Solid Edge part; units mm, degrees
sketch "Sketch1" plane through (0, 0, 0) normal (0, -1, 0) x (1, 0, 0)
  line L0 (0, 0) -> (-45, 0)
  line L1 (-45, 0) -> (-45, -4)
  line L2 (0, -4) -> (-45, -4)
  line L3 (28.2843, -32.2843) -> (0, -4)
  line L4 (30.2843, -30.2843) -> (28.2843, -32.2843)
  line L5 (0, 0) -> (30.2843, -30.2843)
  dimension "D1" = 45
  dimension "D2" = 28.2843
extrude "Protrusion1" add sketch "Sketch1" along normal mid plane 30
sketch "Sketch2" plane through (-15, 0, 0) normal (0, 0, 1) x (1, 0, 0)
  circle A0 centre (-8, 0) radius 7.5
  dimension "D1" = 8
extrude "Cutout1" cut sketch "Sketch2" against normal up to surface (4 mm away)
sketch "Sketch3" plane through (10.6066, 0, -10.6066) normal (0.7071068, 0, 0.7071068) x (0.7071068, 0, -0.7071068)
  circle A0 centre (10.8284, 0) radius 7.5
extrude "Cutout2" cut sketch "Sketch3" against normal up to surface (2.8284 mm away)
properties material "Stainless steel"
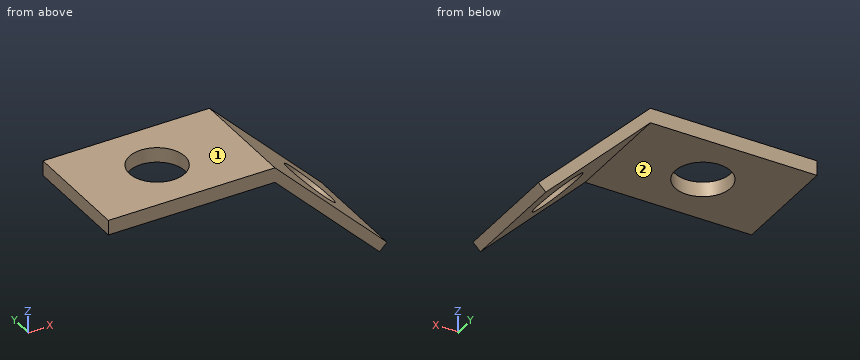
Can you work these out from the model? Positions are in its coordinate system, mm. Face numbers are marked on the shaded views. A direction names the side the tool comes from. Give positions to 0.01 mm unless a question says otherwise; leave off trailing zeros. Order: outer loops, then holes, each group sorted by start corner. A loop starts at its lowest first (then second) coordinate and runs counter-clockwise, first axis right, second up. Notation, with made-up numbers: (89, 55) - (93, 55) arc R32 cw to (93, 92) - close; hole circle Ø4 at (88.25, 38.5). An arc over 180 degrees is marked (long way). Use a Markdown table: item, result. Add a question column.
Q1. On a 3-axis mill with a long thin cutter (end or side, diameter ignored), from which of +Z, -Z, +X, -X, +Y, -Y can I reach the whole of each face in a straight line? I mean the marked faces 1 and 2. Say none if no direction works.
Q2. If we section it at B-B on x = -23: Write out the boundary of the cut face in (y, z).
Q3. Please list where these lines run through material, in increasing order: line 1 along Y through (x, z) = (-23, -2.8); line 2 along Z through (x, y) = (-37.5, 4); line 3 along X through (y, z) = (-5.5, -23.5).
Q4. If we section it at A-A on y = -4: Write out the boundary of the cut face in (x, z).
Q5. I'm going to push flat-ended pins straight in: pin 1 (8 mm diameter, centred on x = -10, y = -11.5, fed in from -Z); pin 2 (3 mm diameter, centred on y = -11, z = -18.5, fed in from -X); pin 3 (4 mm diameter, centred on y = -8, z = -12, fed in from -X). Where does each tip first touch, or does it pass through?
Q6. If we section it at D-D on y = 0: Write out the boundary of the cut face in (x, z).
Q7. If we section it at C-C on y = 11: Write out the boundary of the cut face in (x, z).
Answers follow:
| question | item | result |
|---|---|---|
| 1 | face 1 | +Z, +X, -X, +Y, -Y |
| 1 | face 2 | -Z, -X, +Y, -Y |
| 2 | outline | (-15, -4) - (-7.5, -4) - (-7.5, 0) - (-15, 0) - close; (7.5, -4) - (15, -4) - (15, 0) - (7.5, 0) - close |
| 3 | line 1 | y = -15 to -7.5, 7.5 to 15 |
| 3 | line 2 | z = -4 to 0 |
| 3 | line 3 | x = 20.24 to 23.5 |
| 4 | outline | (-45, -4) - (-29.34, -4) - (-29.34, 0) - (-45, 0) - close; (-16.66, -4) - (0, -4) - (11.78, -15.78) - (13.78, -13.78) - (0, 0) - (-16.66, 0) - close; (20.75, -24.75) - (28.28, -32.28) - (30.28, -30.28) - (22.75, -22.75) - close |
| 5 | pin 1 | stops at z = -4 |
| 5 | pin 2 | stops at x = 13 |
| 5 | pin 3 | stops at x = 6 |
| 6 | outline | (-45, -4) - (-30.5, -4) - (-30.5, 0) - (-45, 0) - close; (-15.5, -4) - (0, -4) - (10.96, -14.96) - (12.96, -12.96) - (0, 0) - (-15.5, 0) - close; (21.57, -25.57) - (28.28, -32.28) - (30.28, -30.28) - (23.57, -23.57) - close |
| 7 | outline | (-45, -4) - (0, -4) - (28.28, -32.28) - (30.28, -30.28) - (0, 0) - (-45, 0) - close |
